Design review of the part built by this model. Coordinates are the model's own, in mm. Face numbers are marked on the shaded views. A direction names the side the tool comes from. Round coordinates to 2 decimals unless told otherwise and drop trailing zeros. Loops run counter-clockwise (first coordinate to the right, second up) from the corner with the lowest first, then second, coordinate; pieces in that order, holes last. Notation, with made-up numbers: (83.5, 34.25) - (108.5, 34.25) arc R15 cw to (108.5, 41.25) - close; hole circle Ø5 at (83.5, 50.5). An arc over 180 degrees is marked (long way). Return JSON: item names as keys, results as strings. Group by question number.
(1) Wall thickness on L1, parallel to Z at x = -40, y = 68.25; L2, parallel to X at y = 54, z = 64; L3, parallel to Z at x = -40, y = 33.5: over which ranges is each line inside the solid? List them lowest first. Write a range as [from, to].
(2) Clearance check with flat-ended pins moving along their axes: pin 1 (2 mm diameter, centred on y = 61, z = 54, fed in from -X); pin 2 (6.5 mm diameter, centred on x = -38.5, z = 37.5, fed in from +Y); pin 3 (4 mm diameter, centred on x = -0.5, z = 60.5, fed in from +Y). State where each tip first meets the part, or that it passes through.
(3) For the marked faces 1, 2 and 3, list the 3-axis set-ups (+Z, -Z, +X, -X, +Y, -Y) from which the entire face can be reached by the end or side of a thin tool; tool diameter is ignored.
(4) We need section A-A, the plane y = 28. Write out the cut boundary in (x, z), and give its area (3 significant figures).
(5) We need section C-C, the plane x = 0. Write out the cut boundary in (y, z).
(6) The part is to be moulded in two halves that separate along Y. For the marked faces 4, 5, 6 and 7, say which applies: pulls with the +Y half, pulls with the -Y half, needs draft (parallel to the pull), parting line crosses it, or undercut.
(7) We need section D-D, the plane y = 50. Write out the cut boundary in (x, z).
(8) We need section B-B, the plane z = 39. Write out the cut boundary in (x, y), and give its area (3 significant figures).
from build123d import *

# Parameters (mm, degrees)
EXTRUDE_1_DEPTH        = 78
PATTERN_LINEAR_1_COUNT = 3
PATTERN_LINEAR_1_PITCH = 23.5
SKETCH_26_W            = 4.5
SKETCH_26_H            = 40
M8X1_257_D             = 6.8
M8X1_257_DEPTH         = 14.41228676


with BuildPart() as part:
    # Эскиз1 → Бобышка-Вытянуть1 (new body)
    with BuildSketch(Plane.XY):
        with BuildLine():
            Line((-64.5, 0), (64.5, 0))
            Line((64.5, 0), (64.5, 15))
            Line((64.5, 15), (49.5, 15))
            Line((49.5, 15), (49.5, 71))
            Line((49.5, 71), (32, 71))
            ThreePointArc((32, 71), (0, 86), (-32, 71))
            Line((-32, 71), (-49.5, 71))
            Line((-49.5, 71), (-49.5, 46))
            Line((-49.5, 46), (-32.465366161, 46))
            ThreePointArc((-32.465366161, 46), (32.5, 44.5), (-32.465366161, 43))
            Line((-32.465366161, 43), (-49.5, 43))
            Line((-49.5, 43), (-49.5, 15))
            Line((-49.5, 15), (-64.5, 15))
            Line((-64.5, 15), (-64.5, 0))
        make_face()
    extrude(amount=EXTRUDE_1_DEPTH)

    # Эскиз14 → Вырез-Повернуть2 (revolve, cut)
    with BuildSketch(Plane.ZY.offset(40), mode=Mode.PRIVATE) as cut_revolve_2_sk:
        Polygon((55.75, 62), (55.75, 71), (62.5, 71), (62.5, 60.41228676), (58.5, 60.41228676), align=None)
    cut_revolve_2 = revolve(cut_revolve_2_sk.sketch.rotate(Axis((-40, 71, 62.5), (0, -1, 0)), 180), axis=Axis((-40, 71, 62.5), (0, -1, 0)), mode=Mode.SUBTRACT)

    # Линейный массив1: Вырез-Повернуть2 ×3
    with Locations(*[(0, 0, -i * PATTERN_LINEAR_1_PITCH) for i in range(1, PATTERN_LINEAR_1_COUNT)]):
        add(cut_revolve_2, mode=Mode.SUBTRACT)

    # Эскиз24 → Отверстие обработанное метчиком M8x1.254 (revolve, cut)
    with BuildSketch(Plane(origin=(-40, 43, 62.5), x_dir=(0, 0, 1), z_dir=(1, 0, 0))):
        Polygon((0, 0), (0, 27.042926105), (3.4, 25), (3.4, 0), align=None)
    m8x1_254 = revolve(axis=Axis((-40, 49.35, 62.5), (0, -1, 0)), mode=Mode.SUBTRACT)

    # Эскиз26 → Диаметр отверстия Ø9.0 (9)2 (revolve, cut)
    with BuildSketch(Plane(origin=(-40, 46, 62.5), x_dir=(0, 0, -1), z_dir=(1, 0, 0))):
        with Locations((2.25, 20)):
            Rectangle(SKETCH_26_W, SKETCH_26_H)
    hole_wizard_9_0_9_2 = revolve(axis=Axis((-40, 39.65, 62.5), (0, 1, 0)), mode=Mode.SUBTRACT)

    # Отверстие обработанное метчиком M8x1.257
    with Locations(Plane(origin=(0, 60.41228676, 0), x_dir=(1, 0, 0), z_dir=(0, 1, 0))):
        with Locations((-40, -39)):
            Hole(M8X1_257_D / 2, depth=M8X1_257_DEPTH)

    # Зеркальное отражение1: Отверстие обработанное метчиком M8x1.254, Диаметр отверстия Ø9.0 (9)2 across plane
    add(m8x1_254.mirror(Plane.XY.offset(39)), mode=Mode.SUBTRACT)
    add(hole_wizard_9_0_9_2.mirror(Plane.XY.offset(39)), mode=Mode.SUBTRACT)


solid = part.part
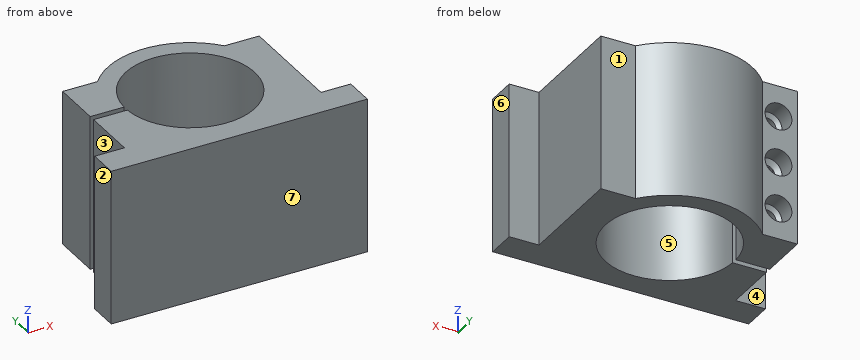
Solutions:
{
 "1": {"L1": "[0, 8.75], [22.25, 32.25], [45.75, 55.75], [69.25, 78]", "L2": "[-49.5, -44.24], [-35.76, -31.08], [31.08, 49.5]", "L3": "[0, 12.1], [18.9, 59.1], [65.9, 78]"},
 "2": {"pin 1": "x = -49.5", "pin 2": "y = 61.2", "pin 3": "y = 86"},
 "3": {"face 1": "+Z, -Z, +X, +Y", "face 2": "+Z, -Z, -X, +Y, -Y", "face 3": "+Z, -Z, -X, +Y"},
 "4": {"outline": "(-49.5, 0) - (-28, 0) - (-28, 78) - (-49.5, 78) - close; (28, 0) - (49.5, 0) - (49.5, 78) - (28, 78) - close; hole circle Ø6.8 at (-40, 15.5); hole circle Ø6.8 at (-40, 62.5)", "area": "3,280 mm^2"},
 "5": {"outline": "(0, 0) - (12, 0) - (12, 78) - (0, 78) - close; (77, 0) - (86, 0) - (86, 78) - (77, 78) - close"},
 "6": {"face 4": "pulls with the +Y half", "face 5": "undercut", "face 6": "needs draft", "face 7": "pulls with the -Y half"},
 "7": {"outline": "(-49.5, 0) - (-32.03, 0) - (-32.03, 78) - (-49.5, 78) - close; (32.03, 0) - (49.5, 0) - (49.5, 78) - (32.03, 78) - close; hole circle Ø9 at (-40, 15.5); hole circle Ø9 at (-40, 62.5); hole circle Ø6.8 at (-40, 39)"},
 "8": {"outline": "(-64.5, 0) - (64.5, 0) - (64.5, 15) - (49.5, 15) - (49.5, 71) - (32, 71) arc R41.63 ccw to (-32, 71) - (-33.25, 71) - (-33.25, 62) - (-36, 60.41) - (-36.6, 60.41) - (-36.6, 46) - (-32.47, 46) arc R32.5 cw (long way) to (-32.47, 43) - (-49.5, 43) - (-49.5, 15) - (-64.5, 15) - close; (-49.5, 46) - (-43.4, 46) - (-43.4, 60.41) - (-44, 60.41) - (-46.75, 62) - (-46.75, 71) - (-49.5, 71) - close", "area": "4,540 mm^2"}
}
